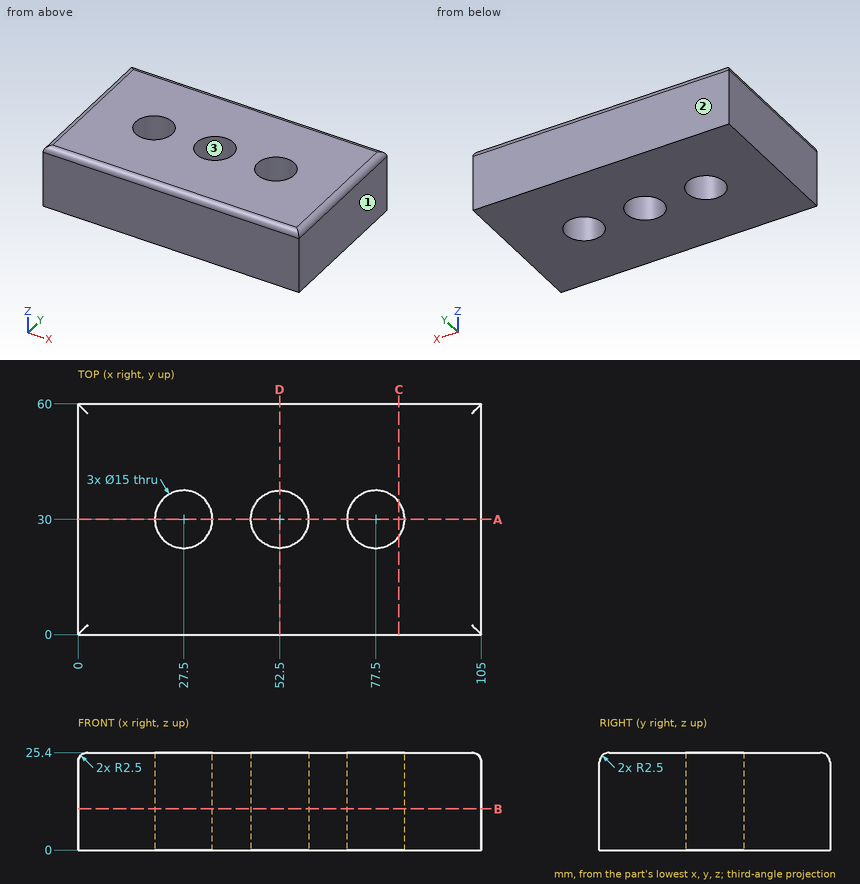
Source: three-view drawing plus pictorial views. Frame: mm from the lowest corner of the part. Round coordinates to 2 decimals unless told otherwise and drop trailing zeros. Loops run counter-clockwise (first coordinate to the right, second up) from the corner with the lowest first, then second, coordinate; pieces in that order, holes last.
1. Section query B-B on z = 10.75. Output: boundary loops of the cut face in (x, y).
2. Section query D-D on x = 52.5. Output: boundary loops of the cut face in (y, z), and give its area (3 significant figures).
3. Section query C-C on x = 83.5. Output: boundary loops of the cut face in (y, z), and give its area (3 significant figures).
4. Ray query, L1, parallel to Y at x = 52.5, z = 9; L2, parallel to X at y = 28.5, z = 19; L3, parallel to X at y = 36.5, z = 9.75. Return the intervals inside material, ascending.
5. Mould query, pull axis Y, two halves, no side actions, for the marked faces 1, 2 and 3. Classes: released by +Y, released by -Y, zero draft, split by the parting line, or undercut.
6. Section query A-A on y = 30. Output: boundary loops of the cut face in (x, z).
Answers below:
1. outline: (0, 0) - (105, 0) - (105, 60) - (0, 60) - close; hole circle Ø15 at (27.5, 30); hole circle Ø15 at (52.5, 30); hole circle Ø15 at (77.5, 30)
2. outline: (0, 0) - (22.5, 0) - (22.5, 25.4) - (2.5, 25.4) arc R2.5 ccw to (0, 22.9) - close; (37.5, 0) - (60, 0) - (60, 22.9) arc R2.5 ccw to (57.5, 25.4) - (37.5, 25.4) - close
2. area: 1,140 mm2
3. outline: (0, 0) - (25.5, 0) - (25.5, 25.4) - (2.5, 25.4) arc R2.5 ccw to (0, 22.9) - close; (34.5, 0) - (60, 0) - (60, 22.9) arc R2.5 ccw to (57.5, 25.4) - (34.5, 25.4) - close
3. area: 1,290 mm2
4. L1: y = 0 to 22.5, 37.5 to 60
4. L2: x = 0 to 20.15, 34.85 to 45.15, 59.85 to 70.15, 84.85 to 105
4. L3: x = 0 to 23.76, 31.24 to 48.76, 56.24 to 73.76, 81.24 to 105
5. face 1: zero draft
5. face 2: released by +Y
5. face 3: undercut
6. outline: (0, 0) - (20, 0) - (20, 25.4) - (2.5, 25.4) arc R2.5 ccw to (0, 22.9) - close; (35, 0) - (45, 0) - (45, 25.4) - (35, 25.4) - close; (60, 0) - (70, 0) - (70, 25.4) - (60, 25.4) - close; (85, 0) - (105, 0) - (105, 22.9) arc R2.5 ccw to (102.5, 25.4) - (85, 25.4) - close
